Here's the drawing with two shaded views (mm, measured from the low corner). I have some questions. Round coordinates to 2 decimals unless told otherwise and drop trailing zeros. Order: outer loops, then holes, each group sorted by start corner. A loop starts at its lowest first (then second) coordinate and runs counter-clockwise, first axis right, second up.
Q1. If we section it at A-A (z = 85): Please give me the cut outline in (x, y), plus the area to 3 significant figures.
Q2. Will these pins go through, and if not, where does the flat tip stop? P1, Ø6, axis at x = 472, z = 97.5, coming from the +Y side (1 decimal); P2, Ø12, axis at x = 117, z = 74, coming from the -Y side; P3, Ø10, axis at x = 492, z = 134, coming from the +Y side.
Q3. If we section it at C-C (x = 69): Please give me the cut outline in (y, z), plus the area to 3 significant figures.
Q4. If I drill on line 1 (X direction, y = 159, z = 106); line 2 (X direction, y = 204.5, z = 24); line 3 (Y direction, x = 75, z = 91.5) (1 decimal), over which ranges is the centre line in solid material (lowest first)?
Q5. If we section it at B-B (y = 810.5): Please give me the cut outline in (x, z), plus the area to 3 significant figures.
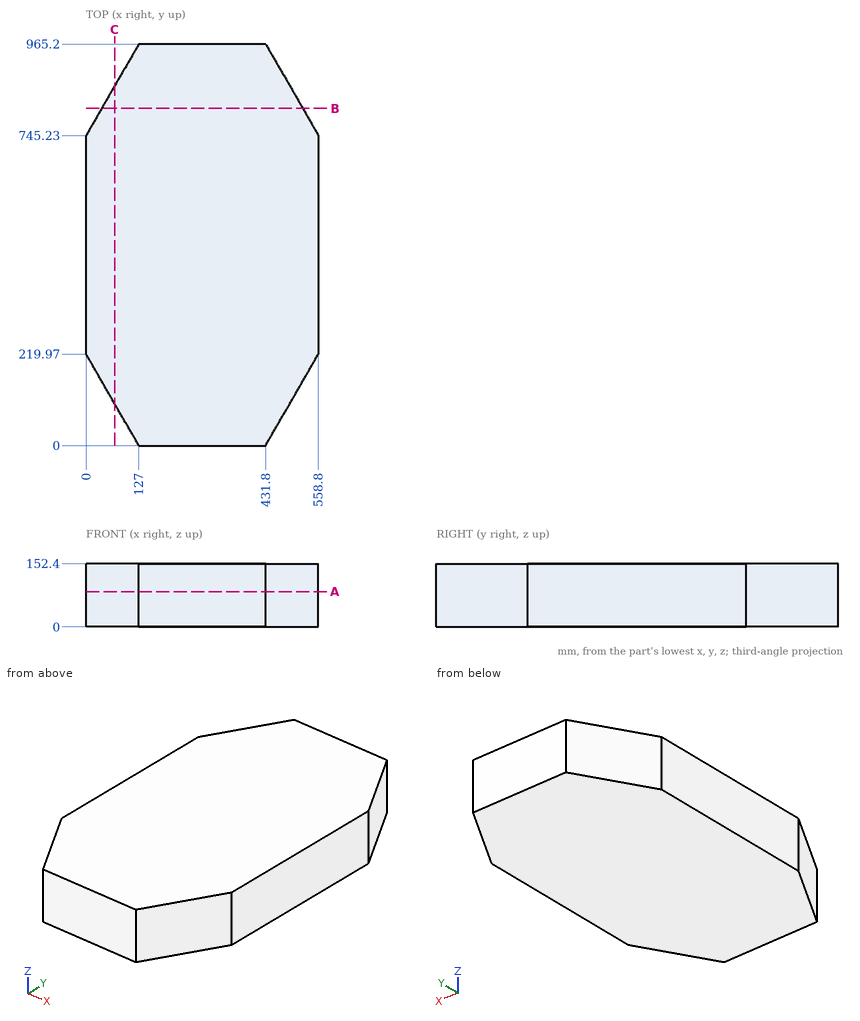
Solution:
1. outline: (0, 219.97) - (127, 0) - (431.8, 0) - (558.8, 219.97) - (558.8, 745.23) - (431.8, 965.2) - (127, 965.2) - (0, 745.23) - close
1. area: 483,000 mm2
2. P1: stops at y = 900.8
2. P2: stops at y = 6.93
2. P3: stops at y = 869.59
3. outline: (100.46, 0) - (864.74, 0) - (864.74, 152.4) - (100.46, 152.4) - close
3. area: 116,000 mm2
4. line 1: x = 35.2 to 523.6
4. line 2: x = 8.93 to 549.87
4. line 3: y = 90.1 to 875.1
5. outline: (37.68, 0) - (521.12, 0) - (521.12, 152.4) - (37.68, 152.4) - close
5. area: 73,700 mm2
